from build123d import *

# Parameters (mm, degrees)
SKETCH2_R          = 3.1115
CUT_EXTRUDE1_DEPTH = 7.62


with BuildPart() as part:
    # Sketch1 → Revolve1 (revolve)
    with BuildSketch(Plane.XY, mode=Mode.PRIVATE) as revolve1_sk:
        with BuildLine():
            Line((37.719, 0), (37.719, 15.24))
            Line((37.719, 15.24), (15.24, 15.24))
            Line((15.24, 15.24), (15.24, 0))
            add(Edge.make_bspline(
                [(15.24, 0), (26.468860477, 6.797265709), (37.719, 0)],
                knots=[0, 0, 0, 1, 1, 1], degree=2))
        make_face()
    revolve(revolve1_sk.sketch.rotate(Axis((0, 0, 0), (0, 1, 0)), 90), axis=Axis((0, 0, 0), (0, 1, 0)))

    # Sketch2 → Cut-Extrude1 (cut)
    with BuildSketch(Plane(origin=(0, 15.24, 0), x_dir=(1, 0, 0), z_dir=(0, 1, 0))):
        with Locations(Location((15.24, -26.396454307, 0), (0, 0, 270))):
            Circle(SKETCH2_R)
        with Locations(Location((-15.24, 26.396454307, 0), (0, 0, 270))):
            Circle(SKETCH2_R)
    extrude(amount=-CUT_EXTRUDE1_DEPTH, mode=Mode.SUBTRACT)


solid = part.part
Verification items for the finished model (mm, model axes). A direction names the side the tool comes from. Round coordinates to 2 decimals unless told otherwise and drop trailing zeros. Loops run counter-clockwise (first coordinate to the right, second up) from the corner with the lowest first, then second, coordinate; pieces in that order, holes last. Notation, with made-up numbers: (7, 37) - (65, 37) arc R16 ccw to (65, 57) - close; hole circle Ø8 at (5, 82.25). An arc over 180 degrees is marked (long way). Answer in a Markdown table with one row per item. Add a question column.
Q1. Section check B-B on y = 4.5. Enter the section's corners in (x, z).
Q2. Release check for a two-part mould opening along Z. For faces 3 (the face through (36.82, 7.73, 8.18)), 4 (the face through (16, 15.24, 1)), 5 (the face through (15, 7.62, 26)) record: pulls with the +Z half, pulls with the -Z half, needs draft (parallel to the pull), parting line crosses it, or undercut.
Q3. Tool access check on faces 1 (the face through (-15.11, 7.51, 1.98)), 2 (the face through (17.864, 11.483, 28.069)). Record the directions out of +Z, -Z, +X, -X, +Y, -Y that give a thin tool (end or side, any length) a straight path to the whole face; none if there is none.
Q4. Material ranges on line 1 (Z direction, x = -14, y = 12.75); line 2 (X direction, y = 3.75, z = 0); line 3 (Z direction, x = -5.5, y = 12.25), recorded low to high.
Q5. Section check A-A on y = 10.5. Enter the section's corners in (x, z), plus the area to 3 significant figures.
Q6. Gauge pin test, flat ends, axial feed: pin 1 (3 mm diameter, centred on x = -14, z = -28, fed in from +Y); pin 2 (10 mm diameter, centred on x = -15.24, z = -26.4, fed in from -Y); pin 3 (6 mm diameter, centred on x = -5.5, z = 24, fed in from -Y) (3 decimals); pin 4 (1.9 mm diameter, centred on x = 14, z = 27.5, fed in from +Y). Record the tip position at first contact, or that the pin passes through.
Found:
| question | item | result |
|---|---|---|
| 1 | outline | circle Ø75.44 at (0, 0); hole circle Ø30.48 at (0, 0) |
| 2 | face 3 | parting line crosses it |
| 2 | face 4 | needs draft |
| 2 | face 5 | undercut |
| 3 | face 1 | +Y, -Y |
| 3 | face 2 | +Y |
| 4 | line 1 | z = -35.02 to -29.25, -23.54 to -6.02, 6.02 to 35.02 |
| 4 | line 2 | x = -37.72 to -15.24, 15.24 to 37.72 |
| 4 | line 3 | z = -37.32 to -14.21, 14.21 to 37.32 |
| 5 | outline | circle Ø75.44 at (0, 0); hole circle Ø6.22 at (-15.24, -26.4); hole circle Ø30.48 at (0, 0); hole circle Ø6.22 at (15.24, 26.4) |
| 5 | area | 3,680 mm² |
| 6 | pin 1 | stops at y = 15.24 |
| 6 | pin 2 | stops at y = 1.22 |
| 6 | pin 3 | stops at y = 2.765 |
| 6 | pin 4 | stops at y = 7.62 |
